Design review of the part built by this model. Coordinates are the model's own, in mm. Coordinates: 2 decimals unless noted, no trailing zeros. Loops run counter-clockwise (first coordinate to the right, second up) from the corner with the lowest first, then second, coordinate; pieces in that order, holes last. Notation, with made-up numbers: (44.25, 39.5) - (101.25, 39.5) arc R26 cw to (101.25, 63.5) - close; hole circle Ø6 at (-1, 38). An arc over 180 degrees is marked (long way). Answer in a Markdown table with one row per item. Add a question column.
(1) We need section B-B, the plane x = -38. Write out the cut boundary in (y, z), plus the area to 3 significant figures.
(2) To check wall thickness, follow L1, parallel to X at y = 0.7, z = 15.5; L2, parallel to Z at x = -4.5, y = 1.6. State the ranges of each line that lie inside material, in increasing order. Write a range as [from, to].
(3) We need section A-A, the plane y = 0.9. Write out the cut boundary in (x, z), plus the area to 3 significant figures.
(4) Clearance check with flat-ended pins moving along their axes: pin 1 (0.6 mm diameter, centred on y = 1, z = -16, fed in from +X); pin 2 (0.6 mm diameter, centred on x = 45, y = 1, fed in from -Z); pin 3 (1 mm diameter, centred on y = 1, z = 16, fed in from -X). State where each tip first meets the part, or that it passes through.
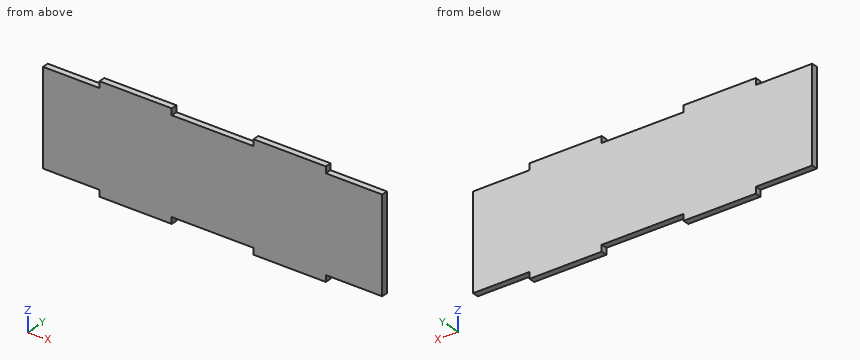
from build123d import *

# Parameters (mm, degrees)
SKETCH_1_W      = 107.9
SKETCH_1_H      = 29.5
EXTRUDE_1_DEPTH = 2
SKETCH_2_W      = 23
SKETCH_2_H      = 2
EXTRUDE_2_DEPTH = 2


with BuildPart() as part:
    # 草图1 → 凸台-拉伸1 (new body)
    with BuildSketch(Plane(origin=(0, 0, 0), x_dir=(1, 0, 0), z_dir=(0, 1, 0))):
        Rectangle(SKETCH_1_W, SKETCH_1_H)
    extrude(amount=EXTRUDE_1_DEPTH)

    # 草图2 → 凸台-拉伸2 (add)
    with BuildSketch(Plane(origin=(0, 2, 0), x_dir=(1, 0, 0), z_dir=(0, 1, 0))):
        with Locations((-24.5, 15.75)):
            Rectangle(SKETCH_2_W, SKETCH_2_H)
        with Locations((24.5, 15.75)):
            Rectangle(SKETCH_2_W, SKETCH_2_H)
        with Locations((24.5, -15.75)):
            Rectangle(SKETCH_2_W, SKETCH_2_H)
        with Locations((-24.5, -15.75)):
            Rectangle(SKETCH_2_W, SKETCH_2_H)
    extrude(amount=-EXTRUDE_2_DEPTH)


solid = part.part
Responses:
| question | item | result |
|---|---|---|
| 1 | outline | (0, -14.75) - (2, -14.75) - (2, 14.75) - (0, 14.75) - close |
| 1 | area | 59.0 mm2 |
| 2 | L1 | x = [-36, -13], [13, 36] |
| 2 | L2 | z = [-14.75, 14.75] |
| 3 | outline | (-53.95, -14.75) - (-36, -14.75) - (-36, -16.75) - (-13, -16.75) - (-13, -14.75) - (13, -14.75) - (13, -16.75) - (36, -16.75) - (36, -14.75) - (53.95, -14.75) - (53.95, 14.75) - (36, 14.75) - (36, 16.75) - (13, 16.75) - (13, 14.75) - (-13, 14.75) - (-13, 16.75) - (-36, 16.75) - (-36, 14.75) - (-53.95, 14.75) - close |
| 3 | area | 3,370 mm2 |
| 4 | pin 1 | stops at x = 36 |
| 4 | pin 2 | stops at z = -14.75 |
| 4 | pin 3 | stops at x = -36 |
